Verification items for the finished model (mm, model axes). A direction names the side the tool comes from. Round coordinates to 2 decimals unless told otherwise and drop trailing zeros. Order: outer loops, then holes, each group sorted by start corner. A loop starts at its lowest first (then second) coordinate and runs counter-clockwise, first axis right, second up. Notation, with made-up numbers: (31.5, -21) -> (79.5, -21) arc R24 ccw to (79.5, 8) -> close; hole circle Ø11 at (-34, -26.75). An arc over 180 degrees is marked (long way). Answer in a Markdown table with one row per item. Add a question column.
```python
from build123d import *

# Parameters (mm, degrees)
BOSS_EXTRUDE1_DEPTH = 50.8
CUT_EXTRUDE1_DEPTH  = 2.27


with BuildPart() as part:
    # Sketch2 → Boss-Extrude1 (new body, symmetric)
    with BuildSketch(Plane(origin=(0, 0, 0), x_dir=(1, 0, 0), z_dir=(0, 1, 0))):
        with BuildLine():
            Line((-5.969, 0), (19.431, 0))
            ThreePointArc((19.431, 0), (19.700407684, -0.111592316), (19.812, -0.381))
            Line((19.812, -0.381), (19.812, -0.889))
            ThreePointArc((19.812, -0.889), (19.700407684, -1.158407684), (19.431, -1.27))
            Line((19.431, -1.27), (1.016, -1.27))
            ThreePointArc((1.016, -1.27), (0.746592316, -1.381592316), (0.635, -1.651))
            Line((0.635, -1.651), (0.635, -3.937))
            ThreePointArc((0.635, -3.937), (0.746592316, -4.206407684), (1.016, -4.318))
            Line((1.016, -4.318), (1.40496875, -4.318))
            ThreePointArc((1.40496875, -4.318), (1.539672592, -4.293392866), (1.656976563, -4.22275))
            ThreePointArc((1.656976563, -4.22275), (3.556, -5.08), (1.656976563, -5.93725))
            ThreePointArc((1.656976563, -5.93725), (1.539672592, -5.866607134), (1.40496875, -5.842))
            Line((1.40496875, -5.842), (-1.40496875, -5.842))
            ThreePointArc((-1.40496875, -5.842), (-1.539672592, -5.866607134), (-1.656976563, -5.93725))
            ThreePointArc((-1.656976563, -5.93725), (-3.556, -5.08), (-1.656976563, -4.22275))
            ThreePointArc((-1.656976563, -4.22275), (-1.539672592, -4.293392866), (-1.40496875, -4.318))
            Line((-1.40496875, -4.318), (-1.016, -4.318))
            ThreePointArc((-1.016, -4.318), (-0.746592316, -4.206407684), (-0.635, -3.937))
            Line((-0.635, -3.937), (-0.635, -1.651))
            ThreePointArc((-0.635, -1.651), (-0.746592316, -1.381592316), (-1.016, -1.27))
            Line((-1.016, -1.27), (-5.969, -1.27))
            ThreePointArc((-5.969, -1.27), (-6.238407684, -1.158407684), (-6.35, -0.889))
            Line((-6.35, -0.889), (-6.35, -0.381))
            ThreePointArc((-6.35, -0.381), (-6.238407684, -0.111592316), (-5.969, 0))
        make_face()
    extrude(amount=BOSS_EXTRUDE1_DEPTH, both=True)

    # Sketch3 → Cut-Extrude1 (cut, through all)
    with BuildSketch(Plane.XY.offset(1.27)):
        with BuildLine():
            Line((11.08075, 2.38125), (12.66825, 2.38125))
            ThreePointArc((12.66825, 2.38125), (15.0495, 0), (12.66825, -2.38125))
            Line((12.66825, -2.38125), (11.08075, -2.38125))
            ThreePointArc((11.08075, -2.38125), (8.6995, 0), (11.08075, 2.38125))
        make_face()
    extrude(amount=-CUT_EXTRUDE1_DEPTH, mode=Mode.SUBTRACT)


solid = part.part
```
1) Cross-section at B-B, the plane x = 2.5. Record the boundary of the cut face in (y, z).
2) Thickness scan on L1, parallel to Z at x = 0.25, y = -32; L2, parallel to Z at x = 15, y = -19; L3, parallel to Z at x = 1, y = 31.5. Record the ranges inside material, lowest first. Write a range as [from, to].
3) Cross-section at D-D, the plane z = 3. Record the boundary of the cut face in (x, y) (3 decimals), and give its area (3 significant figures).
4) Depth check by flat-ended pin: P1, Ø1.8, axis at y = 16.5, z = 2, coming from the -X side; P2, Ø1.4, axis at x = -0.5, y = -25.5, coming from the +Z side; P3, Ø5.5, axis at x = 10, y = 9.5, coming from the +Z side; P4, Ø6, axis at x = -1, y = -37.5, coming from the +Z side. Enter the tip coordinate at first touch or a pass-through.
5) Draft check along Z on faces 1 (the face through (8.7, -0.1, 0.6)), 2 (the face through (0, 1, 5.842)), 3 (the face through (3.555, 0.711, 5.043)). Enter one of: +Z half, -Z half, draft (parallel to the pull), parting line (faces both ways), or undercut.
6) Tool access check on faces 4 (the face through (-0.635, 1, 3)), 5 (the face through (0.635, 1, 3)), 6 (the face through (15.05, 0.05, 0.64)). Record the directions out of +Z, -Z, +X, -X, +Y, -Y that give a thin tool (end or side, any length) a straight path to the whole face; none if there is none.
7) Cross-section at C-C, the plane y = -23.5. Record the boundary of the cut face in (x, z) (3 decimals), and give its area (3 significant figures).
Results below:
| question | item | result |
|---|---|---|
| 1 | outline | (-50.8, 0) -> (50.8, 0) -> (50.8, 1.27) -> (-50.8, 1.27) -> close; (-50.8, 3.94) -> (50.8, 3.94) -> (50.8, 6.22) -> (-50.8, 6.22) -> close |
| 2 | L1 | [0, 5.84] |
| 2 | L2 | [0, 1.27] |
| 2 | L3 | [0, 1.27], [4.32, 5.84] |
| 3 | outline | (-0.635, -50.8) -> (0.635, -50.8) -> (0.635, 50.8) -> (-0.635, 50.8) -> close |
| 3 | area | 129 mm² |
| 4 | P1 | x = -6.29 |
| 4 | P2 | z = 5.84 |
| 4 | P3 | z = 1.27 |
| 4 | P4 | z = 6.22 |
| 5 | face 1 | draft |
| 5 | face 2 | +Z half |
| 5 | face 3 | undercut |
| 6 | face 4 | -X, +Y, -Y |
| 6 | face 5 | +X, +Y, -Y |
| 6 | face 6 | +Z, -Z |
| 7 | outline | (-6.35, 0.381) arc R0.381 ccw to (-5.969, 0) -> (19.431, 0) arc R0.381 ccw to (19.812, 0.381) -> (19.812, 0.889) arc R0.381 ccw to (19.431, 1.27) -> (1.016, 1.27) arc R0.381 cw to (0.635, 1.651) -> (0.635, 3.937) arc R0.381 cw to (1.016, 4.318) -> (1.405, 4.318) arc R0.381 cw to (1.657, 4.223) arc R1.143 ccw (long way) to (1.657, 5.937) arc R0.381 cw to (1.405, 5.842) -> (-1.405, 5.842) arc R0.381 cw to (-1.657, 5.937) arc R1.143 ccw (long way) to (-1.657, 4.223) arc R0.381 cw to (-1.405, 4.318) -> (-1.016, 4.318) arc R0.381 cw to (-0.635, 3.937) -> (-0.635, 1.651) arc R0.381 cw to (-1.016, 1.27) -> (-5.969, 1.27) arc R0.381 ccw to (-6.35, 0.889) -> close |
| 7 | area | 49.5 mm² |
